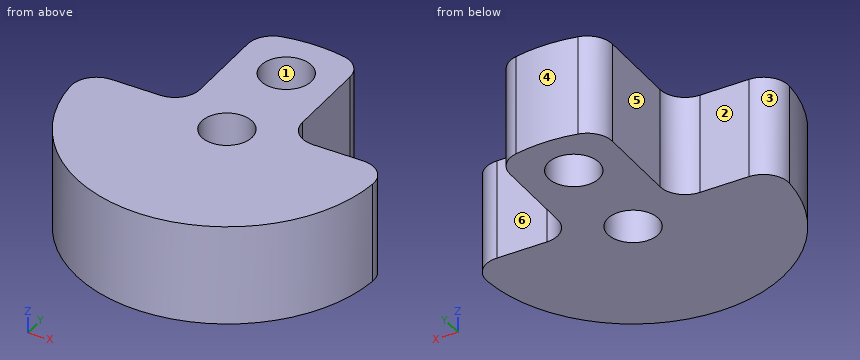
Autodesk Inventor part; units mm, degrees
ref_plane "YZ Plane" through (0, 0, 0) normal (1, 0, 0) x (0, 1, 0)
ref_plane "XZ Plane" through (0, 0, 0) normal (0, 1, 0) x (-1, 0, 0)
ref_plane "XY Plane" through (0, 0, 0) normal (0, 0, 1) x (1, 0, 0)
sketch "Sketch1" plane through (0, 0, 0) normal (0, 0, 1) x (1, 0, 0)
  circle A0 centre (0, 12.7) radius 3.175
  circle A1 centre (-0.0751, 0) radius 3.175
  line L0 (-0.0751, 0) -> (-0.0751, 19.0499)
  line L1 (-0.0751, 3.175) -> (-0.0751, 24.8386)
  line L2 (6.35, 15.5543) -> (6.35, 5.2605)
  line L3 (9.525, 2.0855) -> (15.8376, 2.0855)
  line L4 (-6.5001, 15.5229) -> (-6.5001, 5.2772)
  line L5 (-9.6751, 2.1022) -> (-15.8387, 2.1022)
  arc A2 (-19.0064, -1.2874) -> (19.0051, -1.3074) centre (0, 0) ccw
  arc A3 (3.81, 18.6651) -> (-3.9901, 18.6274) centre (0, 0) ccw
  arc A4 (-3.9901, 18.6274) -> (-6.5001, 15.5229) centre (-3.3251, 15.5229) ccw
  arc A5 (6.35, 15.5543) -> (3.81, 18.6651) centre (3.175, 15.5543) ccw
  arc A6 (6.35, 5.2605) -> (9.525, 2.0855) centre (9.525, 5.2605) ccw
  arc A7 (-9.6751, 2.1022) -> (-6.5001, 5.2772) centre (-9.6751, 5.2772) ccw
  arc A8 (-15.8387, 2.1022) -> (-19.0064, -1.2874) centre (-15.8387, -1.0728) ccw
  arc A9 (19.0051, -1.3074) -> (15.8376, 2.0855) centre (15.8376, -1.0895) ccw
  point P0 (6.35, 17.9605)
  point P1 (6.35, 2.0855)
  point P2 (18.9355, 2.0855)
  point P3 (-6.5001, 2.1022)
  point P4 (-18.9337, 2.1022)
  point P5 (-6.5001, 17.9067)
  dimension "d6" = 6.35
  dimension "d3" = 6.35
  dimension "d11" = 15.875
  dimension "d12" = 3.175
extrude "Extrusion1" add sketch "Sketch1" along normal blind 12.7
properties part number "Crank"
Work out the finished part from the listing and answer in its coordinate system (mm). Face numbers are marked on the shaded views. A direction names the side the tool comes from. Coordinates: 2 decimals unless noted, no trailing zeros. Order: outer loops, then holes, each group sorted by start corner. A loop starts at its lowest first (then second) coordinate and runs counter-clockwise, first axis right, second up. Notation, with made-up numbers: (26, -8) - (44, -8) arc R12 ccw to (44, 8) - close; hole circle Ø9 at (-11.5, 16.25). An arc over 180 degrees is marked (long way). Answer as a JSON object with one key per item and string values.
1. The mould has two halves that part along X. Classify the marked faces 1, 2 and 3: +X half, -X half, draft (parallel to the pull), parting line (faces both ways), or undercut.
Output values:
{"face 1": "undercut", "face 2": "draft", "face 3": "-X half"}
2. Find section D-D on y = 0. Determine the outline of the cut face in (x, z).
Output values:
{"outline": "(-18.83, 0) - (-3.25, 0) - (-3.25, 12.7) - (-18.83, 12.7) - close; (3.1, 0) - (18.82, 0) - (18.82, 12.7) - (3.1, 12.7) - close"}
3. Find section C-C on x = 0. Determine the outline of the cut face in (y, z) (3 decimals), plus the area to 3 significant figures.
Output values:
{"outline": "(-19.05, 0) - (-3.174, 0) - (-3.174, 12.7) - (-19.05, 12.7) - close; (3.174, 0) - (9.525, 0) - (9.525, 12.7) - (3.174, 12.7) - close; (15.875, 0) - (19.05, 0) - (19.05, 12.7) - (15.875, 12.7) - close", "area": "323 mm²"}
4. Consider line 1 (Y direction, x = 0, z = 9) (3 decimals); line 2 (Y direction, x = -1.5, z = 2.5); line 3 (X direction, y = 6.5, z = 12). Determine where each line is inside the solid, lowest interval first.
Output values:
{"line 1": "y = -19.05 to -3.174, 3.174 to 9.525, 15.875 to 19.05", "line 2": "y = -18.99 to -2.84, 2.84 to 9.9, 15.5 to 18.99", "line 3": "x = -6.5 to 6.35"}
5. Each of these flat-tipped pins is pushed along its axis until it touches: P1, Ø1.5, axis at x = 8.5, y = 5, coming from the -Z side; P2, Ø3, axis at x = -13, z = 8.5, coming from the +Y side; P3, Ø7, axis at x = 11.5, z = 8.5, coming from the +Y side; P4, Ø1, axis at y = 10.5, z = 7.5, coming from the -X side. Where does it stop, or does it pass through?
Output values:
{"P1": "passes through", "P2": "stops at y = 2.1", "P3": "stops at y = 2.48", "P4": "stops at x = -6.5"}
6. Find section B-B on y = 12.7. Determine the outline of the cut face in (x, z) (3 decimals), plus the area to 3 significant figures.
Output values:
{"outline": "(-6.5, 0) - (-3.175, 0) - (-3.175, 12.7) - (-6.5, 12.7) - close; (3.175, 0) - (6.35, 0) - (6.35, 12.7) - (3.175, 12.7) - close", "area": "82.6 mm²"}
7. Find section A-A on z = 4.25. Count the separate pieces of the cut face and the enclosed holes in it, plus the area to 3 significant figures.
Output values:
{"separate pieces": "1", "enclosed holes": "2", "area": "797 mm²"}
8. A tool of negligible diameter and unlimited length cuts with its end or side. For the marked faces 4, 5 and 6, from which of +Z, -Z, +X, -X, +Y, -Y can it reach the whole face along a straight path? Write none if from no direction.
Output values:
{"face 4": "+Z, -Z, +Y", "face 5": "+Z, -Z, -X, +Y", "face 6": "+Z, -Z, +X, +Y"}
